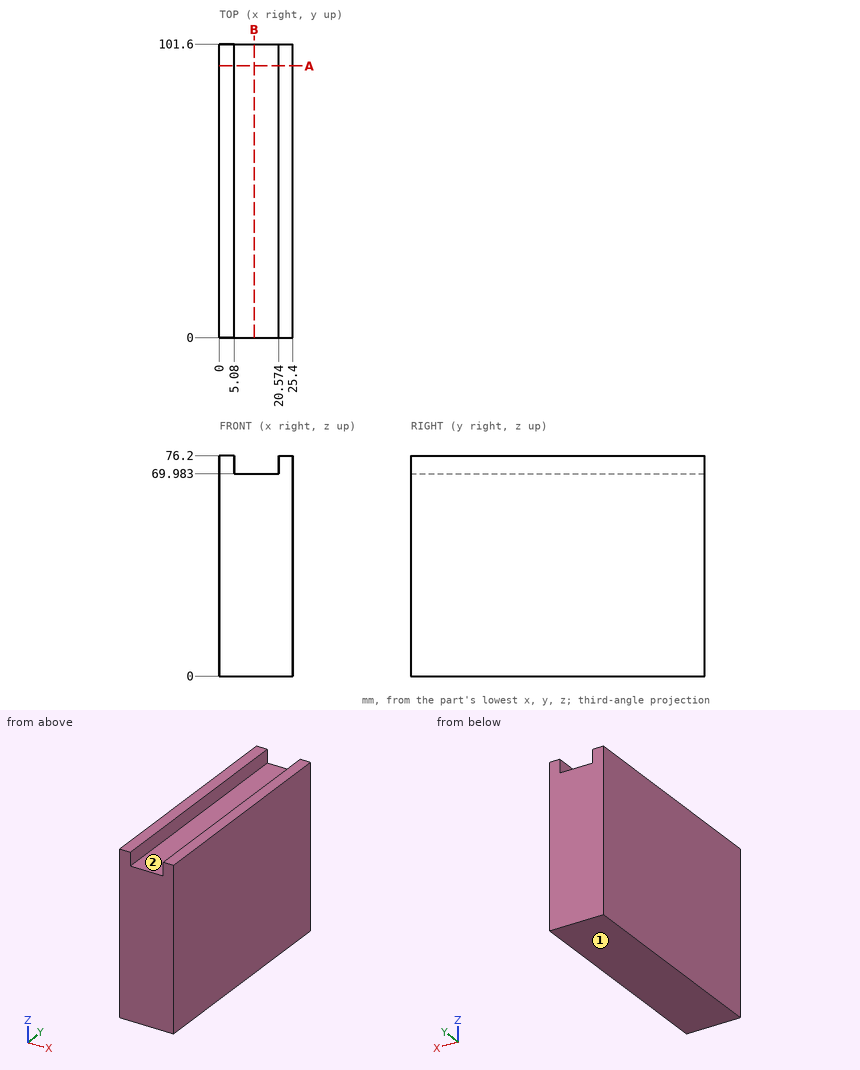
Input: dimensioned drawing with shaded views. Units: mm. Origin: part minimum x, y, z. A direction names the side the tool comes from. Coordinates: 2 decimals unless noted, no trailing zeros. Order: outer loops, then holes, each group sorted by start corner. A loop starts at its lowest first (then second) coordinate and runs counter-clockwise, first axis right, second up.
Item 1: Contact query for a flat-ended pin moving along its axis: P1, Ø7.5, axis at x = 10, y = 39.5, coming from the +Z side. Output: stop coordinate, or through.
Answer:
P1: stops at z = 69.98
Item 2: Material intervals for line 1 along Z through (x, y) = (9.5, 69), sorted ascending.
Answer:
line 1: z = 0 to 69.98
Item 3: Section query B-B (x = 12). Output: boundary loops of the cut face in (y, z), then the cut area to 3 significant figures.
Answer:
outline: (0, 0) - (101.6, 0) - (101.6, 69.98) - (0, 69.98) - close
area: 7,110 mm2
Item 4: Section query A-A (y = 94). Output: boundary loops of the cut face in (x, z).
Answer:
outline: (0, 0) - (25.4, 0) - (25.4, 76.2) - (20.57, 76.2) - (20.57, 69.98) - (5.08, 69.98) - (5.08, 76.2) - (0, 76.2) - close
Item 5: Access query for the marked faces 1 and 2. Directions: +Z, -Z, +X, -X, +Y, -Y. A direction counts if a zero-diameter tool reaches every point of the face in a straight line with its end or side. Return the directions, or none.
Answer:
face 1: -Z, +X, -X, +Y, -Y
face 2: +Z, +Y, -Y
